For this review, take the finished solid that the model builds, in its own axes (mm). A direction names the side the tool comes from. Coordinates: 2 decimals unless noted, no trailing zeros. Order: outer loops, then holes, each group sorted by start corner. A loop starts at its lowest first (then second) coordinate and runs counter-clockwise, first axis right, second up. Notation, with made-up numbers: (9.5, 61.5) -> (48.5, 61.5) arc R20 ccw to (48.5, 75.5) -> close; hole circle Ø10 at (78, 22.5). An arc over 180 degrees is marked (long way). Return JSON: item names as keys, results as strings. Group by question number.
Item 1: Machinability: for faces 5 (the cylindrical face through (-80.476, 29.598, 8.974)), 6 (the cylindrical face through (-94.505, -37.742, 15.496)), which of the approach directions +Z, -Z, +X, -X, +Y, -Y give a long, thin tool a straight path to every point of the face, cutting with its end or side? Answer none if there is none.
Item 2: Take a section at D-D (y = 7.5). Write out the cut boundary in (x, z), then the cut area to 3 significant figures.
Item 3: For line 1 along Y through (x, z) = (-100, 5.5); line 2 along Y through (x, z) = (81.95, 10.75); line 3 along X through (y, z) = (37.5, 8.25), list the stretches that pass through material, from the lowest coordinate up.
Item 4: Insertion check: pin 1 (3 mm diameter, centred on x = -81.95, y = -30.95, fed in from +Z); pin 2 (8 mm diameter, centred on x = 40.5, y = 18.5, fed in from +Z). Each pin has a flat end and moves straight along its axis. Give the tip position at first contact, or say it passes through.
Item 5: Take a section at C-C (x = -70.5). Write out the cut boundary in (y, z).
Item 6: Draft analysis for pull direction X (two halves, no side actions). For faces 1 (the flat face through (112.5, -1, 9)), 2 (the cylindrical face through (86.805, -35.95, 18.207)), 3 (the flat face through (2, 50, 9)), 4 (the flat face through (-102, -35, 12.2)), state which applies: +X half, -X half, draft (parallel to the pull), parting line (faces both ways), or undercut.
Item 7: Take a section at B-B (z = 14.5). Count the separate pieces of the cut face and the enclosed holes in it, then the cut area to 3 significant figures.
Item 8: Take a section at A-A (x = -100). Write out the cut boundary in (y, z), then the cut area to 3 significant figures.
Autodesk Fusion 360 part; units mm, degrees
sketch "Sketch14" plane through (0, 0, 0) normal (0, 0, 1) x (1, 0, 0)
  line L0 (-112.5, -50) -> (112.5, -50)
  line L1 (112.5, -50) -> (112.5, 50)
  line L2 (112.5, 50) -> (-112.5, 50)
  line L3 (-112.5, 50) -> (-112.5, -50)
  line L4 (-112.5, -50) -> (112.5, 50) construction
  line L5 (112.5, -50) -> (-112.5, 50) construction
  dimension "d46" = 225
  dimension "d47" = 100
extrude "Extrude10" add sketch "Sketch14" along normal blind 18.7
sketch "Sketch15" plane through (0, 0, 18.7) normal (0, 0, 1) x (-1, 0, 0)
  line L0 (112.5, -50) -> (112.5, 50)
  line L1 (112.5, 50) -> (-112.5, 50)
  line L2 (-112.5, 50) -> (-112.5, -50)
  line L3 (-112.5, -50) -> (112.5, -50)
  line L4 (80.5859, 35.05) -> (-80.5859, 35.05)
  line L5 (-86.05, 29.5859) -> (-86.05, -29.5859)
  line L6 (-80.5859, -35.05) -> (80.5859, -35.05)
  line L7 (86.05, -29.5859) -> (86.05, 29.5859)
  line L8 (86.05, 35.05) -> (-86.05, -35.05) construction
  line L9 (-86.05, 35.05) -> (86.05, -35.05) construction
  line L10 (0, -40) -> (0, 40) construction
  line L11 (90, 0) -> (-90, 0) construction
  arc A0 (80.5859, -35.05) -> (86.05, -29.5859) centre (84.05, -33.05) ccw
  arc A1 (-86.05, -29.5859) -> (-80.5859, -35.05) centre (-84.05, -33.05) ccw
  arc A2 (-80.5859, 35.05) -> (-86.05, 29.5859) centre (-84.05, 33.05) ccw
  arc A3 (86.05, 29.5859) -> (80.5859, 35.05) centre (84.05, 33.05) ccw
  dimension "d50" = 172.1
  dimension "d51" = 70.1
  dimension "d89" = 8
  dimension "d90" = 2
  dimension "d91" = 2
extrude "Extrude11" cut sketch "Sketch15" against normal blind 1 contours L4 L5 L6 L7 A0 A1 A2 A3
sketch "Sketch16" plane through (0, 0, 18.7) normal (0, 0, 1) x (-1, 0, 0)
  line L0 (86.1, -35.1) -> (86.1, 35.1)
  line L1 (86.1, 35.1) -> (-86.1, 35.1)
  line L2 (-86.1, 35.1) -> (-86.1, -35.1)
  line L3 (-86.1, -35.1) -> (86.1, -35.1)
  circle A0 centre (100, -37.5) radius 5.5
  circle A1 centre (100, 37.5) radius 5.5
  circle A2 centre (-100, -37.5) radius 5.5
  circle A3 centre (-100, 37.5) radius 5.5
  line L4 (112.5, -50) -> (112.5, 50)
  line L5 (-112.5, -50) -> (112.5, -50)
  line L6 (112.5, 50) -> (-112.5, 50)
  line L7 (-112.5, 50) -> (-112.5, -50)
  line L8 (-80.5859, 35.05) -> (80.5859, 35.05)
  line L9 (86.05, 29.5859) -> (86.05, -29.5859)
  line L10 (80.5859, -35.05) -> (-80.5859, -35.05)
  line L11 (-86.05, -29.5859) -> (-86.05, 29.5859)
  line L12 (112.5, -50) -> (112.5, 50)
  line L13 (112.5, 50) -> (-112.5, 50)
  line L14 (-112.5, 50) -> (-112.5, -50)
  line L15 (-112.5, -50) -> (112.5, -50)
  arc A4 (86.05, 29.5859) -> (80.5859, 35.05) centre (84.05, 33.05) ccw
  arc A5 (80.5859, -35.05) -> (86.05, -29.5859) centre (84.05, -33.05) ccw
  arc A6 (-86.05, -29.5859) -> (-80.5859, -35.05) centre (-84.05, -33.05) ccw
  arc A7 (-80.5859, 35.05) -> (-86.05, 29.5859) centre (-84.05, 33.05) ccw
  dimension "d54" = 11
  dimension "d55" = 11
  dimension "d56" = 11
  dimension "d57" = 11
  dimension "d58" = 12.5
  dimension "d59" = 12.5
  dimension "d60" = 12.5
  dimension "d61" = 12.5
  dimension "d62" = 12.5
  dimension "d63" = 12.5
  dimension "d64" = 12.5
  dimension "d65" = 12.5
extrude "Extrude12" cut sketch "Sketch16" against normal blind 6.5 contours A0 | A1 | A2 | A3
sketch "Sketch17" plane through (0, 0, 12.2) normal (0, 0, 1) x (-1, 0, 0)
  circle A0 centre (100, -37.5) radius 5.5
  circle A1 centre (100, -37.5) radius 3
  dimension "d68" = 6
sketch "Sketch18" plane through (0, 0, 12.2) normal (0, 0, 1) x (-1, 0, 0)
  circle A0 centre (-100, -37.5) radius 5.5
  circle A1 centre (-100, -37.5) radius 3
  dimension "d69" = 6
sketch "Sketch19" plane through (0, 0, 12.2) normal (0, 0, 1) x (-1, 0, 0)
  circle A0 centre (-100, 37.5) radius 5.5
  circle A1 centre (-100, 37.5) radius 3
  dimension "d70" = 6
sketch "Sketch20" plane through (0, 0, 12.2) normal (0, 0, 1) x (-1, 0, 0)
  circle A0 centre (100, 37.5) radius 5.5
  circle A1 centre (100, 37.5) radius 3
  dimension "d71" = 6
extrude "Extrude13" cut sketch "Sketch18" sketch "Sketch17" sketch "Sketch20" sketch "Sketch19" along normal up to surface contours A1 of sketch 2 contours A1 of sketch 3 contours A1 of sketch 4 contours A1 end surface through (0, 0, 0) normal (0, 0, -1) offset 0
sketch "Sketch21" plane through (0, 0, 17.7) normal (0, 0, 1) x (-1, 0, 0)
  line L0 (86.05, -29.5859) -> (86.05, 29.5859)
  line L1 (80.5859, 35.05) -> (-80.5859, 35.05)
  line L2 (-86.05, 29.5859) -> (-86.05, -29.5859)
  line L3 (-80.5859, -35.05) -> (80.5859, -35.05)
  circle A0 centre (81.95, -30.95) radius 2
  circle A1 centre (-81.95, -30.95) radius 2
  circle A2 centre (-81.95, 30.95) radius 2
  circle A3 centre (81.95, 30.95) radius 2
  arc A4 (86.05, 29.5859) -> (80.5859, 35.05) centre (84.05, 33.05) ccw
  arc A5 (-80.5859, 35.05) -> (-86.05, 29.5859) centre (-84.05, 33.05) ccw
  arc A6 (-86.05, -29.5859) -> (-80.5859, -35.05) centre (-84.05, -33.05) ccw
  arc A7 (80.5859, -35.05) -> (86.05, -29.5859) centre (84.05, -33.05) ccw
  dimension "d74" = 4
  dimension "d75" = 4
  dimension "d76" = 4
  dimension "d77" = 4
  dimension "d78" = 4.1
  dimension "d79" = 4.1
  dimension "d80" = 4.1
  dimension "d81" = 4.1
  dimension "d82" = 4.1
  dimension "d83" = 4.1
  dimension "d84" = 4.1
  dimension "d85" = 4.1
extrude "Extrude14" cut sketch "Sketch21" against normal blind 20 contours A0 | A1 | A2 | A3
thread "Thread1"
sketch "Sketch4" plane through (0, 0, 2) normal (0, 0, 1) x (-1, 0, 0)
  circle A0 centre (-75, -25) radius 5.5
  circle A1 centre (-75, -25) radius 3.1
  dimension "d20" = 6.2
sketch "Sketch5" plane through (0, 0, 2) normal (0, 0, 1) x (-1, 0, 0)
  circle A0 centre (-75, 25) radius 5.5
  circle A1 centre (-75, 25) radius 3.1
  dimension "d21" = 6.2
sketch "Sketch6" plane through (0, 0, 2) normal (0, 0, 1) x (-1, 0, 0)
  circle A0 centre (75, 25) radius 5.5
  circle A1 centre (75, 25) radius 3.1
  dimension "d22" = 6.2
Findings below:
{
 "1": {"face 5": "+Z, -Z", "face 6": "+Z"},
 "2": {"outline": "(-112.5, 0) -> (112.5, 0) -> (112.5, 18.7) -> (86.05, 18.7) -> (86.05, 17.7) -> (-86.05, 17.7) -> (-86.05, 18.7) -> (-112.5, 18.7) -> close", "area": "4,040 mm2"},
 "3": {"line 1": "y = -50 to -40.5, -34.5 to 34.5, 40.5 to 50", "line 2": "y = -50 to -32.95, -28.95 to 28.95, 32.95 to 50", "line 3": "x = -112.5 to -103, -97 to 97, 103 to 112.5"},
 "4": {"pin 1": "passes through", "pin 2": "stops at z = 17.7"},
 "5": {"outline": "(-50, 0) -> (50, 0) -> (50, 18.7) -> (35.05, 18.7) -> (35.05, 17.7) -> (-35.05, 17.7) -> (-35.05, 18.7) -> (-50, 18.7) -> close"},
 "6": {"face 1": "+X half", "face 2": "undercut", "face 3": "draft", "face 4": "undercut"},
 "7": {"separate pieces": "1", "enclosed holes": "8", "area": "22,100 mm2"},
 "8": {"outline": "(-50, 0) -> (-40.5, 0) -> (-40.5, 12.2) -> (-43, 12.2) -> (-43, 18.7) -> (-50, 18.7) -> close; (-34.5, 0) -> (34.5, 0) -> (34.5, 12.2) -> (32, 12.2) -> (32, 18.7) -> (-32, 18.7) -> (-32, 12.2) -> (-34.5, 12.2) -> close; (40.5, 0) -> (50, 0) -> (50, 18.7) -> (43, 18.7) -> (43, 12.2) -> (40.5, 12.2) -> close", "area": "1,580 mm2"}
}
